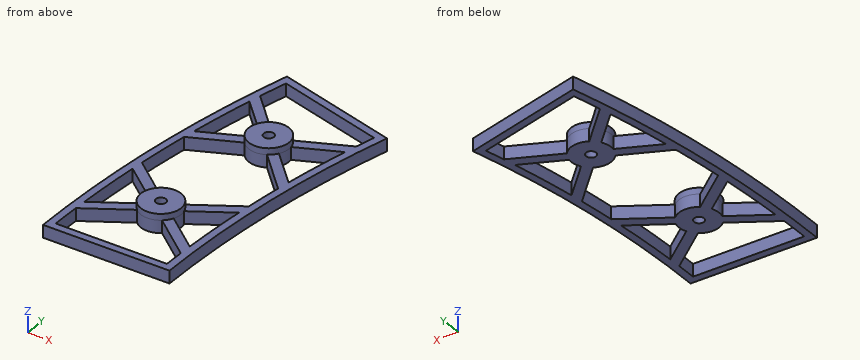
from build123d import *

# Parameters (mm, degrees)
SKETCH_R      = 2
PAD_DEPTH     = 5
SKETCH001_R   = 8
SKETCH001_R_2 = 2.024761308
SKETCH001_R_3 = 8.0000008109
SKETCH001_R_4 = 2.000001045
PAD001_DEPTH  = 2.5


with BuildPart() as part:
    # Sketch → Pad (new body)
    with BuildSketch(Plane.XY):
        with BuildLine():
            ThreePointArc((15.7593053413, 119.7038083599), (3.9567516146, 60.3683639018), (0, 0))
            Line((50, 0), (0, 0))
            ThreePointArc((64.0555966558, 106.7628561048), (53.5289946833, 53.8420542908), (50, 0))
            Line((64.0555966558, 106.7628561048), (15.7593053413, 119.7038083599))
        make_face()
        with Locations((26.0657280113, 30.5184572631)):
            Circle(SKETCH_R, mode=Mode.SUBTRACT)
        with Locations((33.0381072416, 83.4789354772)):
            Circle(SKETCH_R, mode=Mode.SUBTRACT)
        with BuildLine():
            Line((47, 3), (3, 3))
            ThreePointArc((3.2176751035, 14.4566952549), (3.0731243146, 8.7290261724), (3, 3))
            Line((20.4562148001, 24.8146548881), (3.2176751035, 14.4566952549))
            ThreePointArc((20.4562148001, 24.8146548881), (25.5076762214, 22.537944861), (30.8268339618, 24.0894705522))
            Line((30.8268339618, 24.0894705522), (47.1317951682, 10.8859733054))
            ThreePointArc((47.1317951682, 10.8859733054), (47.0471860802, 6.9432993707), (47, 3))
        make_face(mode=Mode.SUBTRACT)
        with BuildLine():
            Line((60.3813620416, 104.6415357612), (17.8806256849, 116.0295737457))
            ThreePointArc((17.8806256849, 116.0295737457), (16.4684772655, 110.4768334411), (15.1256727632, 104.9069174527))
            Line((29.0959862421, 90.4402343521), (15.1256727632, 104.9069174527))
            ThreePointArc((39.3009266424, 88.4565948824), (34.5645792047, 91.3319529448), (29.0959862421, 90.4402343521))
            Line((39.3009266424, 88.4565948824), (58.4676263177, 96.9901593805))
            ThreePointArc((60.3813620416, 104.6415357612), (59.4063393174, 100.820388402), (58.4676263177, 96.9901593805))
        make_face(mode=Mode.SUBTRACT)
        with BuildLine():
            ThreePointArc((18.7873404966, 33.8388601281), (18.0852156092, 31.076509053), (18.3960625004, 28.2433240909))
            Line((18.3960625004, 28.2433240909), (3.3926933694, 19.2283904273))
            ThreePointArc((5.1846193956, 44.8541264837), (4.1095496121, 32.053782821), (3.3926933694, 19.2283904273))
            Line((18.7873404966, 33.8388601281), (5.1846193956, 44.8541264837))
        make_face(mode=Mode.SUBTRACT)
        with BuildLine():
            Line((21.3046220608, 36.9474439739), (5.6753960094, 49.6037416816))
            ThreePointArc((8.4029238656, 70.3213726134), (6.9213768313, 59.9780635876), (5.6753960094, 49.6037416816))
            Line((26.7752878409, 78.5012760721), (8.4029238656, 70.3213726134))
            ThreePointArc((26.7752878409, 78.5012760721), (31.5116352786, 75.6259180097), (36.9802282412, 76.5176366024))
            Line((36.9802282412, 76.5176366024), (51.5545531991, 61.4254813054))
            ThreePointArc((51.5545531991, 61.4254813054), (50.5439225691, 54.2350464901), (49.6590953227, 47.0280493451))
            Line((31.6752412226, 36.222259638), (49.6590953227, 47.0280493451))
            ThreePointArc((31.6752412226, 36.222259638), (26.6237798013, 38.4989696651), (21.3046220608, 36.9474439739))
        make_face(mode=Mode.SUBTRACT)
        with BuildLine():
            Line((33.344115526, 27.198054398), (47.2935739714, 15.9020056772))
            ThreePointArc((49.121202926, 42.0383173978), (48.0013333151, 28.9845703161), (47.2935739714, 15.9020056772))
            Line((33.7353935222, 32.7935904352), (49.121202926, 42.0383173978))
            ThreePointArc((33.344115526, 27.198054398), (34.0462404134, 29.9604054731), (33.7353935222, 32.7935904352))
        make_face(mode=Mode.SUBTRACT)
        with BuildLine():
            Line((39.8575874425, 79.2962700842), (52.3264266993, 66.384409056))
            ThreePointArc((57.3256479332, 92.1031727317), (54.6232740747, 79.2832040754), (52.3264266993, 66.384409056))
            Line((40.9278732147, 84.8024130518), (57.3256479332, 92.1031727317))
            ThreePointArc((39.8575874425, 79.2962700842), (40.8911247092, 81.9524635142), (40.9278732147, 84.8024130518))
        make_face(mode=Mode.SUBTRACT)
        with BuildLine():
            Line((25.1483412686, 82.1554579027), (9.1581609295, 75.0361709325))
            ThreePointArc((14.0597218383, 100.25251579), (11.4326959844, 87.6786019965), (9.1581609295, 75.0361709325))
            Line((26.2186270408, 87.6616008703), (14.0597218383, 100.25251579))
            ThreePointArc((26.2186270408, 87.6616008703), (25.1850897741, 85.0054074403), (25.1483412686, 82.1554579027))
        make_face(mode=Mode.SUBTRACT)
    extrude(amount=PAD_DEPTH)

    # Sketch001 (on Face44 of Pad) → Pad001 (join)
    with BuildSketch(Plane.XY.offset(5)):
        with Locations((33.0381072416, 83.4789354772)):
            Circle(SKETCH001_R)
        with Locations((33.04052, 83.454292)):
            Circle(SKETCH001_R_2, mode=Mode.SUBTRACT)
        with Locations((26.065727, 30.518457)):
            Circle(SKETCH001_R_3)
        with Locations((26.065727, 30.518457)):
            Circle(SKETCH001_R_4, mode=Mode.SUBTRACT)
    extrude(amount=PAD001_DEPTH)


solid = part.part
Source: CAD feature listing. Evaluate the final solid. Frame: model axes, mm. Give positions to 0.01 mm unless a question says otherwise; leave off trailing zeros. Write each loop counter-clockwise with the first axis right and the second up, starting at its lowest first coordinate (ties: lowest second). Pieces come first, ordered by that corner, then holes. Notation, with made-up numbers: (51.25, 30.25) - (105.25, 30.25) arc R19 cw to (105.25, 48.25) - close; hole circle Ø10 at (-4.75, 48.25). An arc over 180 degrees is marked (long way). Write item = value, one per line. Start each with the question number.
Q1. Cut plane B-B, the plane x = 45. Return loops of the section in (y, z).
Q2. Cut plane D-D, the plane z = 3.25. Give the number of separate pieces and of enclosed holes in the cut face, then the cut area to 3 significant figures.
Q3. Cut plane C-C, the plane y = 108. Return loops of the section in (x, z).
Q4. Cut plane A-A, the plane y = 73.5. Return loops of the section in (x, z).
Q5. Material intervals for probe 1 along X at (y, z) = (90.5, 3.75); probe 2 along Y at (x, z) = (34.5, 3.25) (3 decimals); probe 3 along X at (y, z) = (82.5, 2), sorted ascending.
Q6. Pin query (flat end, axial travel): pin 1 Ø2.5 at (x, y) = (33.04, 83.45) entering from -Z; pin 2 Ø1.5 at (y, z) = (89.5, 3.5) entering from +X; pin 3 Ø10 at (x, y) = (54.5, 78.5) entering from +Z; pin 4 Ø2.5 at (x, z) = (26, 3) entering from +Y. Return the tip coordinate at first contact, or that it passes through.
Computed values:
q1.outline = (0, 0) - (3, 0) - (3, 5) - (0, 5) - close; (12.61, 0) - (17.76, 0) - (17.76, 5) - (12.61, 5) - close; (39.56, 0) - (44.23, 0) - (44.23, 5) - (39.56, 5) - close; (68.21, 0) - (73.97, 0) - (73.97, 5) - (68.21, 5) - close; (86.62, 0) - (90.99, 0) - (90.99, 5) - (86.62, 5) - close; (108.76, 0) - (111.87, 0) - (111.87, 5) - (108.76, 5) - close
q2.separate_pieces = 1
q2.enclosed_holes = 9
q2.area = 1,940 mm²
q3.outline = (12.79, 0) - (15.86, 0) - (15.86, 5) - (12.79, 5) - close; (47.85, 0) - (59.44, 0) - (59.44, 5) - (47.85, 5) - close
q4.outline = (5.88, 0) - (15.54, 0) - (15.54, 5) - (5.88, 5) - close; (39.89, 0) - (45.45, 0) - (45.45, 5) - (39.89, 5) - close; (53.54, 0) - (56.6, 0) - (56.6, 5) - (53.54, 5) - close
q5.probe_1 = 8.94 to 11.99, 23.48 to 29.04, 29.2 to 36.87, 43.89 to 53.72, 56.96 to 60.05
q5.probe_2 = 0 to 3, 21.115 to 26.262, 33.253 to 37.92, 75.614 to 82.114, 84.844 to 91.344, 111.576 to 114.682
q5.probe_3 = 7.42 to 10.46, 25.1 to 31.29, 34.78 to 40.98, 55.26 to 58.33
q6.pin_1 = through
q6.pin_2 = 59.99
q6.pin_3 = 5
q6.pin_4 = 117.29
